The model under review builds one solid part; all positions refer to its coordinate system, in mm. Coordinates: 2 decimals unless noted, no trailing zeros. Write each loop counter-clockwise with the first axis right and the second up, starting at its lowest first coordinate (ties: lowest second). Pieces come first, ordered by that corner, then holes. Notation, with made-up numbers: M 30.25,28 L 40.25,28 A6 cw 40.25,33 Z; hole C 76.25,82.5 d11. An arc over 180 degrees is marked long. Answer as a JSON object with one key per item and string values.
```python
from build123d import *

# Parameters (mm, degrees)
F2_R      = 25
F3_DEPTH  = 45.001
F3_FACE_R = 25
F4_DEPTH  = 45.001


with BuildPart() as f1:
    # F0 (on Top) → F1 (revolve)
    with BuildSketch(Plane.XY):
        with BuildLine():
            Line((0, 0), (0, -45))
            ThreePointArc((0, -45), (45, 0), (0, 45))
            Line((0, 45), (0, 0))
        make_face()
    revolve(axis=Axis((0, 29.846651, 0), (0, 1, 0)))

    # F2 (on Top) → F3 (cut, through all)
    with BuildSketch(Plane.XY):
        Circle(F2_R)
    extrude(amount=-F3_DEPTH, mode=Mode.SUBTRACT)

    # F3_face (on face) → F4 (cut, through all)
    with BuildSketch(Plane(origin=(0, 0, 0), x_dir=(1, 0, 0), z_dir=(0, 0, -1))):
        Circle(F3_FACE_R)
    extrude(amount=-F4_DEPTH, mode=Mode.SUBTRACT)


solid = f1.part
```
(1) Add section D-D on x = 26.5. Give the boundary of the cut face in (y, z), and give its area (3 significant figures).
Results list:
{"outline": "C 0,0 d72.74", "area": "4,160 mm²"}
(2) For pin 1 Ø6 at (x, z) = (13.5, 30.5) entering from +Y; pin 2 Ø1.5 at (y, z) = (-30.5, 29.5) entering from +X; pin 3 Ø1.5 at (y, z) = (-26, 22.5) entering from -X, all flat-tipped, find the tip position at first contact; note any pin that passes through.
Results list:
{"pin 1": "y = 33.22", "pin 2": "x = 16.96", "pin 3": "x = -29.9"}
(3) Add section A-A on y = 0. Give the boundary of the cut face in (x, z).
Results list:
{"outline": "M -25,-37.42 L -25,37.42 A45 ccw Z; M 25,-37.42 A45 ccw 25,37.42 Z"}
(4) Add section C-C on z = -18. Give the boundary of the cut face in (x, y).
Results list:
{"outline": "C 0,0 d82.49; hole C 0,0 d50"}
(5) Wall thickness on line 1 along Y through (x, z) = (0, -1); line 2 along Y through (x, z) = (0, 11.5); line 3 along X through (y, z) = (0, 19): over which ranges is each line inside the solid? List them lowest first. Write a range as from..to.
Results list:
{"line 1": "-44.99..-25, 25..44.99", "line 2": "-43.51..-25, 25..43.51", "line 3": "-40.79..-25, 25..40.79"}
